```python
from build123d import *

# Parameters (mm, degrees)
BOSS_EXTRUDE1_DEPTH  = 20.5
BOSS_EXTRUDE2_START  = 5
BOSS_EXTRUDE2_DEPTH  = 5
BOSS_EXTRUDE3_DEPTH  = 5
FILLET1_R            = 2
SKETCH8_R            = 2.9
CUT_EXTRUDE4_DEPTH   = 5
FILLET1_OF_MIRROR3_R = 2
FILLET2_R            = 2.5
SKETCH9_R            = 3.5
CUT_EXTRUDE5_DEPTH   = 50
SKETCH17_R           = 4
CUT_EXTRUDE8_DEPTH   = 50


with BuildPart() as part:
    # Sketch1 → Boss-Extrude1 (new, symmetric)
    with BuildSketch(Plane(origin=(0, 0, 0), x_dir=(1, 0, 0), z_dir=(0, 1, 0))):
        with BuildLine():
            Line((-15.4, 0), (-17, 0))
            ThreePointArc((-17, 0), (0, 17), (17, 0))
            Line((17, 0), (15.4, 0))
            ThreePointArc((15.4, 0), (0, 15.4), (-15.4, 0))
        make_face()
    extrude(amount=BOSS_EXTRUDE1_DEPTH, both=True)

    # Sketch6 → Boss-Extrude2 (add)
    with BuildSketch(Plane(origin=(0, 20.5, 0), x_dir=(1, 0, 0), z_dir=(0, 1, 0)).offset(BOSS_EXTRUDE2_START)):
        with BuildLine():
            Line((-17, 0), (-7, 0))
            ThreePointArc((-7, 0), (0, 7), (7, 0))
            Line((7, 0), (17, 0))
            ThreePointArc((17, 0), (0, 17), (-17, 0))
        make_face()
    boss_extrude2 = extrude(amount=-BOSS_EXTRUDE2_DEPTH)

    # Mirror1: Boss-Extrude2 across plane
    add(boss_extrude2.mirror(Plane.ZX))

    # Sketch7 → Boss-Extrude3 (add, symmetric)
    with BuildSketch(Plane(origin=(0, 0, 0), x_dir=(1, 0, 0), z_dir=(0, 1, 0))):
        with BuildLine():
            Line((-17, 0), (-27, 0))
            Line((-27, 0), (-27, 5))
            Line((-27, 5), (-16.248076809, 5))
            ThreePointArc((-16.248076809, 5), (-16.810968231, 2.528111374), (-17, 0))
        make_face()
    boss_extrude3 = extrude(amount=BOSS_EXTRUDE3_DEPTH, both=True)

    # Fillet1
    fillet1_edges = [part.edges().sort_by_distance(p)[0] for p in [
        (-16.810968231, -5, -2.528111374),
        (-16.248076809, 0, -5),
        (-16.810968231, 5, -2.528111374),
    ]]
    fillet(fillet1_edges, radius=FILLET1_R)

    # Sketch8 → Cut-Extrude4 (cut, symmetric)
    with BuildSketch(Plane(origin=(0, 0, -5), x_dir=(-1, 0, 0), z_dir=(0, 0, -1))):
        with Locations((23.436686237, 0)):
            Circle(SKETCH8_R)
    cut_extrude4 = extrude(amount=CUT_EXTRUDE4_DEPTH, both=True, mode=Mode.SUBTRACT)

    # Mirror3: Boss-Extrude3, Cut-Extrude4 across plane
    add(boss_extrude3.mirror(Plane(origin=(0, 0, 0), x_dir=(0, 0, 1), z_dir=(1, 0, 0))))
    add(cut_extrude4.mirror(Plane(origin=(0, 0, 0), x_dir=(0, 0, 1), z_dir=(1, 0, 0))), mode=Mode.SUBTRACT)

    # Fillet1 of Mirror3
    fillet1_of_mirror3_edges = [part.edges().sort_by_distance(p)[0] for p in [
        (16.810968231, -5, -2.528111374),
        (16.248076809, 0, -5),
        (16.810968231, 5, -2.528111374),
    ]]
    fillet(fillet1_of_mirror3_edges, radius=FILLET1_OF_MIRROR3_R)

    # Fillet2
    fillet2_edges = [part.edges().sort_by_distance(p)[0] for p in [
        (-27, -5, -2.5),
        (-27, 5, -2.5),
        (27, 5, -2.5),
        (27, -5, -2.5),
    ]]
    fillet(fillet2_edges, radius=FILLET2_R)

    # Sketch9 → Cut-Extrude5 (cut)
    with BuildSketch(Plane(origin=(0, 0, 0), x_dir=(0, 0, -1), z_dir=(1, 0, 0))):
        with Locations(Location((8.5, -13, 0), (0, 0, 180))):
            Circle(SKETCH9_R)
    extrude(amount=CUT_EXTRUDE5_DEPTH, mode=Mode.SUBTRACT)

    # Sketch17 → Cut-Extrude8 (cut)
    with BuildSketch(Plane(origin=(0, 0, 0), x_dir=(0, -1, 0), z_dir=(-0.5000000000000011, 0, 0.8660254037844379))):
        with Locations(Location((-13, 1.722431864, 0), (0, 0, 90))):
            Circle(SKETCH17_R)
    extrude(amount=-CUT_EXTRUDE8_DEPTH, mode=Mode.SUBTRACT)


solid = part.part
```
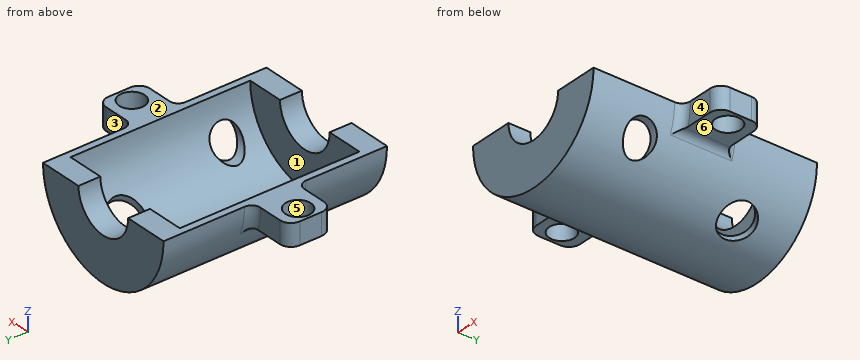
The listing builds one solid part. Answer for the finished solid, in the listing's coordinates (mm). Face numbers are marked on the shaded views. A direction names the side the tool comes from. Give positions to 0.01 mm unless a question says otherwise; leave off trailing zeros. Order: outer loops, then holes, each group sorted by start corner. A loop starts at its lowest first (then second) coordinate and runs counter-clockwise, first axis right, second up.
1) Find section C-C on y = 16. Write down the section's boundary in (x, z).
Reported:
outline: (-17, 0) arc R17 ccw to (7.69, -15.16) - (6.89, -13.77) arc R15.4 cw to (-15.4, 0) - close; (11.17, -10.6) - (12, -12.04) arc R17 ccw to (17, 0) - (15.4, 0) arc R15.4 cw to start
2) For the marked faces 1 and 2, determine the directions among +Z, -Z, +X, -X, +Y, -Y from which every point of the face is accessible in a straight line to the end or side of a thin tool.
Reported:
face 1: +Z
face 2: +Z, +X, -X, +Y, -Y
3) Given P1, Ø1, axis at y = 7, z = -13.5, coming from the +X side; P2, Ø4, axis at x = 20.5, z = -2, coming from the -Y side; P3, Ø6.5, axis at x = -23.44, y = 0, coming from the -Z side, each flat-ended and moving along its own axis, determine where each tip first touches the part or whether it passes through.
Reported:
P1: stops at x = 10.95
P2: stops at y = -5.04
P3: stops at z = -5
4) Find section A-A on y = 0. Write down the section's boundary in (x, z).
Reported:
outline: (-27, -5) - (-26.34, -5) - (-26.34, 0) - (-27, 0) - close; (-20.54, -5) - (-17.66, -5) arc R2 cw to (-15.8, -6.26) arc R17 ccw to (15.8, -6.26) arc R2 cw to (17.66, -5) - (20.54, -5) - (20.54, 0) - (15.4, 0) arc R15.4 cw to (-15.4, 0) - (-20.54, 0) - close; (26.34, -5) - (27, -5) - (27, 0) - (26.34, 0) - close
5) Find section B-B on x = 0. Write down the section's boundary in (y, z).
Reported:
outline: (-25.5, -17) - (25.5, -17) - (25.5, -7) - (20.5, -7) - (20.5, -15.4) - (-20.5, -15.4) - (-20.5, -7) - (-25.5, -7) - close
6) Find section D-D on z = -3.25. Give the number of separate pieces and of enclosed holes in the cut face, then the cut area to 3 significant figures.
Reported:
separate pieces: 2
enclosed holes: 2
area: 495 mm2
7) Determine the mould class of the marked faces 3, 4, 5 and 6 for opening direction Y: pulls with the +Y half, pulls with the -Y half, needs draft (parallel to the pull), parting line crosses it, or undercut.
Reported:
face 3: pulls with the +Y half
face 4: pulls with the -Y half
face 5: undercut
face 6: needs draft
8) Consider line 1 along Y through (x, z) = (12, -8); line 2 along Y through (x, z) = (14, -8.5); line 3 along X through (y, z) = (19, -11.25). Determine where each line is inside the solid, lowest interval first.
Reported:
line 1: y = -25.5 to -20.5, 20.5 to 25.5
line 2: y = -25.5 to -16.5, -9.5 to 25.5
line 3: x = -12.75 to -10.52, 10.52 to 12.75
